Answer from the drawing. Dimensions are ordinates in mm from the lowest x, y and z of the part. A direction names the side the tool comes from. Coordinates: 2 decimals unless noted, no trailing zeros. Order: outer loops, then holes, each group sorted by start corner. A loop starts at its lowest first (then second) coordinate and runs counter-clockwise, first axis right, second up. Notation, with made-up numbers: M 7,-9 L 63,-9 A16 cw 63,2 Z; hole C -16.75,52 d7. An arc over 180 degrees is marked long. Write each question's results on one line, items separated by ' | '.
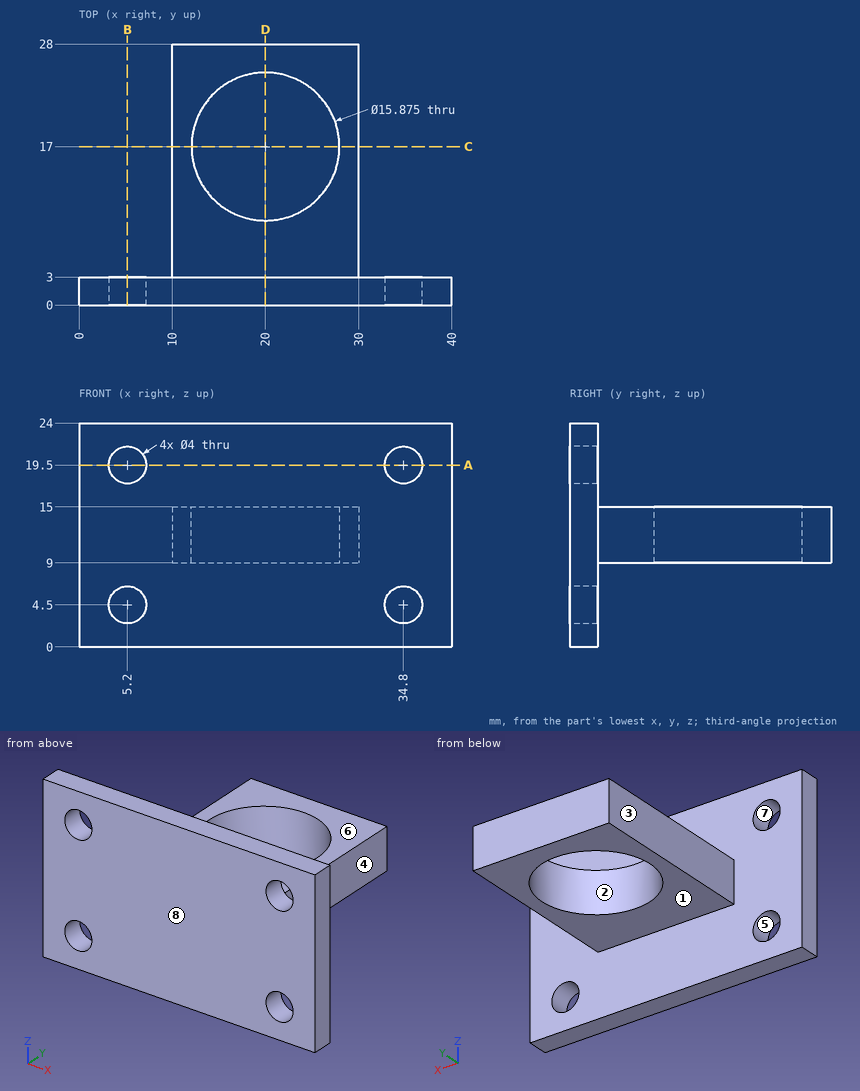
(1) The mould has two halves that part along Z. Classify the marked faces 5, 6, 7 and 8: pulls with the +Z half, pulls with the -Z half, needs draft (parallel to the pull), parting line crosses it, or undercut.
Conclusion:
face 5: undercut | face 6: pulls with the +Z half | face 7: undercut | face 8: needs draft
(2) For the marked faces 1, 2, 3 and 4, determine the directions among +Z, -Z, +X, -X, +Y, -Y from which every point of the face is accessible in a straight line to the end or side of a thin tool.
Conclusion:
face 1: -Z, +X, -X, +Y | face 2: +Z, -Z | face 3: +Z, -Z, -X, +Y | face 4: +Z, -Z, +X, +Y
(3) Given pin 1 (1.5 mm diameter, centred on y = 5, z = 20, fed in from -X); pin 2 (5 mm diameter, centred on x = 5.2, z = 19.5, fed in from +Y); pin 3 (3 mm diameter, centred on y = 10.5, z = 11, fed in from +X); pin 4 (6.5 mm diameter, centred on y = 18, z = 13.5, fed in from -X), each flat-ended and moving along its own axis, determine where each tip first touches the part or whether it passes through.
Conclusion:
pin 1: through | pin 2: y = 3 | pin 3: x = 30 | pin 4: x = 10
(4) The part is cut by section B-B, the plane x = 5.2. Write down the section's boundary in (y, z), then the cut area to 3 significant figures.
Conclusion:
outline: M 0,0 L 3,0 L 3,2.5 L 0,2.5 Z; M 0,6.5 L 3,6.5 L 3,17.5 L 0,17.5 Z; M 0,21.5 L 3,21.5 L 3,24 L 0,24 Z | area: 48.0 mm²
(5) The part is cut by section A-A, the plane z = 19.5. Write down the section's boundary in (x, y).
Conclusion:
outline: M 0,0 L 3.2,0 L 3.2,3 L 0,3 Z; M 7.2,0 L 32.8,0 L 32.8,3 L 7.2,3 Z; M 36.8,0 L 40,0 L 40,3 L 36.8,3 Z
(6) Straight lines are drawn through the part: line 1 (Z direction, x = 5.2, y = 2.05); line 2 (X direction, y = 0.8, z = 4.5); line 3 (Y direction, x = 20, z = 10.9). For each, find the intervals that lie inside material, in ascending order.
Conclusion:
line 1: 0 to 2.5, 6.5 to 17.5, 21.5 to 24 | line 2: 0 to 3.2, 7.2 to 32.8, 36.8 to 40 | line 3: 0 to 9.06, 24.94 to 28
(7) The part is cut by section C-C, the plane y = 17. Write down the section's boundary in (x, z).
Conclusion:
outline: M 10,9 L 12.06,9 L 12.06,15 L 10,15 Z; M 27.94,9 L 30,9 L 30,15 L 27.94,15 Z
(8) The part is cut by section D-D, the plane x = 20. Write down the section's boundary in (y, z).
Conclusion:
outline: M 0,0 L 3,0 L 3,9 L 9.06,9 L 9.06,15 L 3,15 L 3,24 L 0,24 Z; M 24.94,9 L 28,9 L 28,15 L 24.94,15 Z
